Geometry: final body of the model. Coordinates: model frame, mm. Face numbers are marked on the shaded views. A direction names the side the tool comes from. Give positions to 0.01 mm unless a question says otherwise; leave off trailing zeros. Loops run counter-clockwise (first coordinate to the right, second up) from the corner with the lowest first, then second, coordinate; pieces in that order, holes last.
1. Section D-D, the plane z = -28. Output: boundary loops of the cut face in (x, y).
2. Access query for the marked faces 1, 2 and 3. Directions: +Z, -Z, +X, -X, +Y, -Y. A direction counts if a zero-diameter tool reaches every point of the face in a straight line with its end or side. Return the directions, or none.
3. Section B-B, the plane x = -98.5. Output: boundary loops of the cut face in (y, z), then the cut area to 3 significant figures.
4. First-contact query: P1, Ø10.5, axis at x = -59.15, z = -7.38, coming from the +Y side; P2, Ø11, axis at y = 12, z = 11, coming from the -X side; P3, Ø10, axis at y = 26, z = -7, coming from the +X side; P4, Ø4, axis at y = 5, z = 1, coming from the -X side. Flat tips, straight axial feed; report the tip coordinate or a pass-through.
5. Section C-C, the plane y = 5.85. Output: boundary loops of the cut face in (x, z), then the cut area to 3 significant figures.
6. Section A-A, the plane x = -115. Output: boundary loops of the cut face in (y, z).
7. Draft query along Z for the marked faces 4, 5, 6 and 7. Return one class per face: +Z half, -Z half, draft (parallel to the pull), parting line (faces both ways), or undercut.
8. Material intervals for line 1 along Y through (x, z) = (-107, 4); line 2 along Z through (x, y) = (-71, 20); line 3 along Z through (x, y) = (-113, 34), sorted ascending.
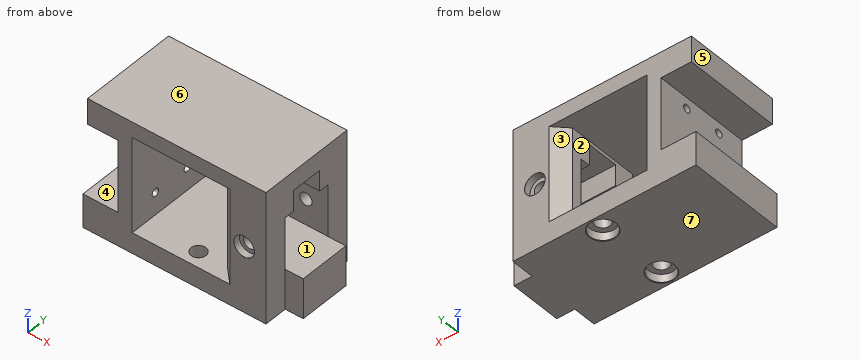
from build123d import *

# Parameters (mm, degrees)
SALIENTE_EXTRUIR1_DEPTH                     = 38
CROQUIS2_W                                  = 32.911764705
CROQUIS2_H                                  = 37
CORTAR_EXTRUIR1_DEPTH                       = 38
CROQUIS3_R                                  = 1.5
CORTAR_EXTRUIR3_DEPTH                       = 10
CROQUIS5_W                                  = 13.588235295
CROQUIS5_H                                  = 38
CORTAR_EXTRUIR4_DEPTH                       = 1
CROQUIS8_W                                  = 20
CROQUIS8_H                                  = 20
CORTAR_EXTRUIR5_DEPTH                       = 8
CROQUIS10_W                                 = 8
CROQUIS10_H                                 = 12
CORTAR_EXTRUIR7_DEPTH                       = 10
CROQUIS11_W                                 = 10
CROQUIS11_H                                 = 38
CORTAR_EXTRUIR8_DEPTH                       = 1.8
CROQUIS13_W                                 = 49
CROQUIS13_H                                 = 38
SALIENTE_EXTRUIR2_DEPTH                     = 12
CROQUIS15_W                                 = 71
CROQUIS15_H                                 = 38
SALIENTE_EXTRUIR3_DEPTH                     = 2
REFRENTADO_PARA_TORNILLO_CON_CABEZA_2_COUNT = 2
REFRENTADO_PARA_TORNILLO_CON_CABEZA_2_PITCH = 26.31900454
CROQUIS18_W                                 = 19
CROQUIS18_H                                 = 8
CORTAR_EXTRUIR9_DEPTH                       = 0.16
CROQUIS19_W                                 = 19
CROQUIS19_H                                 = 8
CORTAR_EXTRUIR10_DEPTH                      = 0.16
CROQUIS20_W                                 = 19
CROQUIS20_H                                 = 12.32
CORTAR_EXTRUIR11_DEPTH                      = 0.1
CHAFL_N3_SIZE                               = 5
CROQUIS26_W                                 = 15.5
CROQUIS26_H                                 = 20
SALIENTE_EXTRUIR4_DEPTH                     = 7


with BuildPart() as part:
    # Croquis1 → Saliente-Extruir1 (new body)
    with BuildSketch(Plane(origin=(0, 0, 0), x_dir=(1, 0, 0), z_dir=(0, 1, 0))):
        Polygon((-121.647058824, 30.882352941), (-62.647058824, 30.882352941), (-62.647058824, -18.117647059), (-121.647058824, -18.117647059), (-121.647058824, -7.117647059), (-108.058823529, -7.117647059), (-108.058823529, 19.882352941), (-121.647058824, 19.882352941), align=None)
    extrude(amount=SALIENTE_EXTRUIR1_DEPTH)

    # Croquis2 → Cortar-Extruir1 (cut)
    with BuildSketch(Plane(origin=(0, 38, 0), x_dir=(1, 0, 0), z_dir=(0, 1, 0))):
        with Locations((-86.102941176, 6.382352941)):
            Rectangle(CROQUIS2_W, CROQUIS2_H)
    extrude(amount=-CORTAR_EXTRUIR1_DEPTH, mode=Mode.SUBTRACT)

    # Croquis3 → Cortar-Extruir3 (cut)
    with BuildSketch(Plane(origin=(-102.558823529, 0, 0), x_dir=(0, 0, -1), z_dir=(1, 0, 0))):
        with Locations((16.132352941, 10.875)):
            Circle(CROQUIS3_R)
        with Locations((16.132352941, 25.875)):
            Circle(CROQUIS3_R)
        with Locations((-3.867647059, 10.875)):
            Circle(CROQUIS3_R)
        with Locations((-3.867647059, 25.875)):
            Circle(CROQUIS3_R)
    extrude(amount=-CORTAR_EXTRUIR3_DEPTH, mode=Mode.SUBTRACT)

    # Croquis5 → Cortar-Extruir4 (cut)
    with BuildSketch(Plane(origin=(0, 0, 7.117647059), x_dir=(-1, 0, 0), z_dir=(0, 0, -1))):
        with Locations((114.852941177, 19)):
            Rectangle(CROQUIS5_W, CROQUIS5_H)
    extrude(amount=-CORTAR_EXTRUIR4_DEPTH, mode=Mode.SUBTRACT)

    # Croquis8 → Cortar-Extruir5 (cut)
    with BuildSketch(Plane(origin=(-62.647058824, 0, 0), x_dir=(0, 0, -1), z_dir=(1, 0, 0))):
        with Locations((7.382352941, 19)):
            Rectangle(CROQUIS8_W, CROQUIS8_H)
    extrude(amount=-CORTAR_EXTRUIR5_DEPTH, mode=Mode.SUBTRACT)

    # Croquis10 → Cortar-Extruir7 (cut)
    with BuildSketch(Plane(origin=(-62.647058824, 0, 0), x_dir=(0, 0, -1), z_dir=(1, 0, 0))):
        with Locations((-6.617647059, 19)):
            Rectangle(CROQUIS10_W, CROQUIS10_H)
    extrude(amount=-CORTAR_EXTRUIR7_DEPTH, mode=Mode.SUBTRACT)

    # Croquis11 → Cortar-Extruir8 (cut)
    with BuildSketch(Plane.ZY.offset(121.647058824)):
        with Locations((13.117647059, 19)):
            Rectangle(CROQUIS11_W, CROQUIS11_H)
    extrude(amount=-CORTAR_EXTRUIR8_DEPTH, mode=Mode.SUBTRACT)

    # Croquis13 → Saliente-Extruir2 (add)
    with BuildSketch(Plane(origin=(-62.647058824, 0, 0), x_dir=(0, 0, -1), z_dir=(1, 0, 0))):
        with Locations((6.382352941, 19)):
            Rectangle(CROQUIS13_W, CROQUIS13_H)
        Polygon((17.382352941, 9), (17.382352941, 29), (-2.617647059, 29), (-2.617647059, 25), (-10.617647059, 25), (-10.617647059, 13), (-2.617647059, 13), (-2.617647059, 9), align=None, mode=Mode.SUBTRACT)
    extrude(amount=SALIENTE_EXTRUIR2_DEPTH)

    # Croquis15 → Saliente-Extruir3 (add)
    with BuildSketch(Plane(origin=(0, 0, -30.882352941), x_dir=(-1, 0, 0), z_dir=(0, 0, -1))):
        with Locations((86.147058824, 19)):
            Rectangle(CROQUIS15_W, CROQUIS15_H)
    extrude(amount=SALIENTE_EXTRUIR3_DEPTH)

    # Croquis17 → Refrentado para tornillo con cabeza plan (revolve, cut)
    with BuildSketch(Plane(origin=(-81.647058824, 5.85, -32.882352941), x_dir=(0, 1, 0), z_dir=(1, 0, 0))):
        Polygon((0, 0), (0, 21.742495795), (2.9, 20), (2.9, 3.3), (5, 3.3), (5, 0.2), (5.2, 0), align=None)
    refrentado_para_tornillo_con_cabeza_plan = revolve(axis=Axis((-81.647058824, 5.85, -39.232352941), (0, 0, 1)), mode=Mode.SUBTRACT)

    # Refrentado para tornillo con cabeza  2: Refrentado para tornillo con cabeza plan ×2
    with Locations(*[Vector(0.037995358, 0.999277916, 0) * (i * REFRENTADO_PARA_TORNILLO_CON_CABEZA_2_PITCH) for i in range(1, REFRENTADO_PARA_TORNILLO_CON_CABEZA_2_COUNT)]):
        add(refrentado_para_tornillo_con_cabeza_plan, mode=Mode.SUBTRACT)

    # Croquis18 → Cortar-Extruir9 (cut)
    with BuildSketch(Plane(origin=(0, 13, 0), x_dir=(1, 0, 0), z_dir=(0, 1, 0))):
        with Locations((-60.147058824, -6.617647059)):
            Rectangle(CROQUIS18_W, CROQUIS18_H)
    extrude(amount=-CORTAR_EXTRUIR9_DEPTH, mode=Mode.SUBTRACT)

    # Croquis19 → Cortar-Extruir10 (cut)
    with BuildSketch(Plane(origin=(0, 25, 0), x_dir=(-1, 0, 0), z_dir=(0, -1, 0))):
        with Locations((60.147058824, -6.617647059)):
            Rectangle(CROQUIS19_W, CROQUIS19_H)
    extrude(amount=-CORTAR_EXTRUIR10_DEPTH, mode=Mode.SUBTRACT)

    # Croquis20 → Cortar-Extruir11 (cut)
    with BuildSketch(Plane(origin=(0, 0, 10.617647059), x_dir=(-1, 0, 0), z_dir=(0, 0, -1))):
        with Locations((60.147058824, 19)):
            Rectangle(CROQUIS20_W, CROQUIS20_H)
    extrude(amount=-CORTAR_EXTRUIR11_DEPTH, mode=Mode.SUBTRACT)

    # Croquis23 → Refrentado para tornillo con cabeza  3 (revolve, cut)
    with BuildSketch(Plane(origin=(-59.147058824, 0, -7.332227312), x_dir=(0, 0, -1), z_dir=(1, 0, 0))):
        Polygon((0, 0), (0, 21.442065486), (2.4, 20), (2.4, 2.6), (4, 2.6), (4, 0.025), (4.025, 0), align=None)
    revolve(axis=Axis((-59.147058824, -6.35, -7.332227312), (0, 1, 0)), mode=Mode.SUBTRACT)

    # Croquis25 → Refrentado para tornillo con cabeza  4 (revolve, cut)
    with BuildSketch(Plane(origin=(-59.147058824, 38, -7.382352941), x_dir=(0, 0, 1), z_dir=(1, 0, 0))):
        Polygon((0, 0), (0, 21.442065486), (2.4, 20), (2.4, 2.6), (4, 2.6), (4, 0.025), (4.025, 0), align=None)
    revolve(axis=Axis((-59.147058824, 44.35, -7.382352941), (0, -1, 0)), mode=Mode.SUBTRACT)

    # Chaflán3
    chafl_n3_edges = [part.edges().sort_by_distance(p)[0] for p in [
        (-69.647058824, 0, -6.382352941),
        (-69.647058824, 38, -6.382352941),
    ]]
    chamfer(chafl_n3_edges, length=CHAFL_N3_SIZE)

    # Croquis26 → Saliente-Extruir4 (add)
    with BuildSketch(Plane(origin=(-50.647058824, 0, 0), x_dir=(0, 0, -1), z_dir=(1, 0, 0))):
        with Locations((25.132352941, 19)):
            Rectangle(CROQUIS26_W, CROQUIS26_H)
    extrude(amount=SALIENTE_EXTRUIR4_DEPTH)


solid = part.part
Answers below:
1. outline: (-121.65, 0) - (-50.65, 0) - (-50.65, 9) - (-43.65, 9) - (-43.65, 29) - (-50.65, 29) - (-50.65, 38) - (-121.65, 38) - close; hole circle Ø5.8 at (-81.65, 5.85); hole circle Ø5.8 at (-80.65, 32.15)
2. face 1: +X
2. face 2: +Y, -Y
2. face 3: +Y
3. outline: (0, -32.88) - (38, -32.88) - (38, -24.88) - (0, -24.88) - close; (0, 12.12) - (38, 12.12) - (38, 18.12) - (0, 18.12) - close
3. area: 532 mm2
4. P1: stops at y = 38
4. P2: stops at x = -119.85
4. P3: stops at x = -50.65
4. P4: stops at x = -108.06
5. outline: (-121.65, -32.88) - (-86.85, -32.88) - (-86.65, -32.68) - (-86.65, -29.58) - (-84.55, -29.58) - (-84.55, -24.88) - (-102.56, -24.88) - (-102.56, 12.12) - (-69.65, 12.12) - (-69.65, -24.88) - (-78.75, -24.88) - (-78.75, -29.58) - (-76.65, -29.58) - (-76.65, -32.68) - (-76.45, -32.88) - (-50.65, -32.88) - (-50.65, 18.12) - (-119.85, 18.12) - (-119.85, 8.12) - (-108.06, 8.12) - (-108.06, -19.88) - (-121.65, -19.88) - close; hole circle Ø4.8 at (-59.15, -7.33)
5. area: 1,930 mm2
6. outline: (0, -32.88) - (38, -32.88) - (38, -19.88) - (0, -19.88) - close; (0, 8.12) - (38, 8.12) - (38, 18.12) - (0, 18.12) - close
7. face 4: undercut
7. face 5: draft
7. face 6: +Z half
7. face 7: -Z half
8. line 1: y = 0 to 9.38, 12.37 to 24.38, 27.37 to 38
8. line 2: z = -32.88 to -24.88, 12.12 to 18.12
8. line 3: z = -32.88 to -19.88, 8.12 to 18.12
